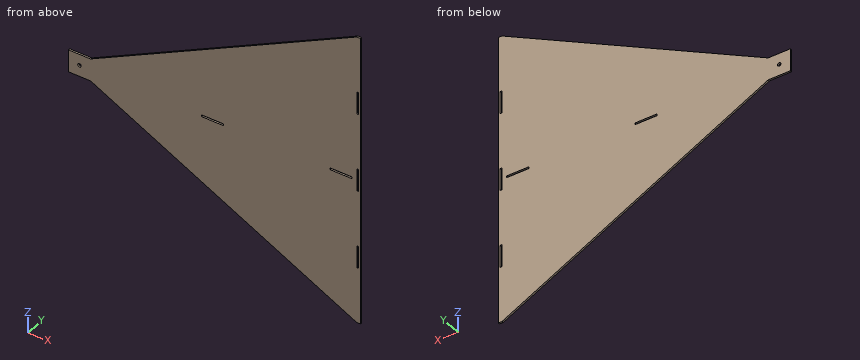
Autodesk Inventor part; units mm, degrees
ref_plane "YZ Plane" through (0, 0, 0) normal (1, 0, 0) x (0, 1, 0)
ref_plane "XZ Plane" through (0, 0, 0) normal (0, 1, 0) x (-1, 0, 0)
ref_plane "XY Plane" through (0, 0, 0) normal (0, 0, 1) x (1, 0, 0)
sketch "Sketch1" plane through (0, 0, 0) normal (0, 1, 0) x (-1, 0, 0)
  line L0 (0, 260) -> (0, -260)
  line L1 (520, 0) -> (0, 260)
  line L2 (0, -260) -> (520, 0)
  point P0 (0, 0)
  dimension "d1" = 260
  dimension "d2" = 520
extrude "Extrusion1" add sketch "Sketch1" along normal blind 3.175
sketch "Sketch2" plane through (0, 3.175, 0) normal (0, 1, 0) x (1, 0, 0)
  circle A0 centre (-500, 0) radius 3.175
  point P0 (0, 0)
  dimension "d6" = 6.35
extrude "Extrusion2" cut sketch "Sketch2" against normal blind 3.175
sketch "Sketch3" plane through (0, 3.175, 0) normal (0, 1, 0) x (1, 0, 0)
  circle A0 centre (-500, 0) radius 3.175
  line L0 (-500, 0) -> (-480, 0)
  line L1 (-480, 0) -> (-480, -20)
  line L2 (-480, -20) -> (-480, 20)
  line L3 (0, 260) -> (-520, 0)
  line L4 (-480, 20) -> (-520, 0)
  line L5 (-520, 0) -> (-480, -20)
  line L6 (-520, 0) -> (0, -260)
  point P0 (0, 0)
extrude "Extrusion3" cut sketch "Sketch3" against normal blind 3.175
sketch "Sketch4" plane through (0, 3.175, 0) normal (0, 1, 0) x (1, 0, 0)
  line L0 (-480, -20) -> (-480, 20)
  line L1 (-480, -20) -> (-520, -20)
  line L2 (-520, -20) -> (-520, 20)
  line L3 (-520, 20) -> (-480, 20)
  point P0 (0, 0)
  dimension "d11" = 40
extrude "Extrusion4" add sketch "Sketch4" against normal blind 3.175
sketch "Sketch5" plane through (0, 3.175, 0) normal (0, 1, 0) x (1, 0, 0)
  circle A0 centre (-500, 0) radius 3.175
  point P0 (0, 0)
  dimension "d15" = 6.35
extrude "Extrusion5" cut sketch "Sketch5" against normal blind 3.175
sketch "Sketch6" plane through (0, 3.175, 0) normal (0, 1, 0) x (1, 0, 0)
  line L0 (-480, -20) -> (0, -260)
  line L1 (0, -260) -> (50, -260)
  line L2 (50, -260) -> (50, 260)
  line L3 (50, 260) -> (0, 260)
  line L4 (0, 260) -> (0, -260)
  point P0 (0, 0)
extrude "Extrusion6" add sketch "Sketch6" against normal blind 3.175
sketch "Sketch8" plane through (0, 3.175, 0) normal (0, 1, 0) x (1, 0, 0)
  line L0 (0, 260) -> (-480, 20)
  line L1 (-480, -20) -> (0, -260)
  line L2 (3.175, -20) -> (0, -20)
  line L3 (0, -20) -> (0, 20)
  line L4 (0, -20) -> (3.2, -20)
  line L5 (0, 20) -> (3.2, 20)
  line L6 (3.2, 20) -> (3.2, -20)
  line L7 (3.2, 160) -> (3.2, 120)
  line L8 (3.2, 120) -> (0, 120)
  line L9 (0, 120) -> (0, 160)
  line L10 (0, 160) -> (3.2, 160)
  line L11 (3.2, -160) -> (3.2, -120)
  line L12 (3.2, -120) -> (0, -120)
  line L13 (0, -120) -> (0, -160)
  line L14 (0, -160) -> (3.2, -160)
  point P0 (0, 0)
  dimension "d23" = 3.2
  dimension "d24" = 3.2
  dimension "d27" = 40
extrude "Extrusion7" cut sketch "Sketch8" against normal blind 10
sketch "Sketch9" plane through (0, 3.175, 0) normal (0, 1, 0) x (1, 0, 0)
  line L0 (3.2, -120) -> (3.2, -160)
  line L1 (6.4, -260) -> (6.4, 260)
  line L2 (0, 260) -> (50, 260)
  line L3 (6.4, 260) -> (50, 260)
  line L4 (50, 260) -> (50, -260)
  line L5 (50, -260) -> (6.4, -260)
  point P0 (0, 0)
extrude "Extrusion8" cut sketch "Sketch9" against normal blind 10
sketch "Sketch10" plane through (0, 3.175, 0) normal (0, 1, 0) x (1, 0, 0)
  line L0 (-520, 20) -> (-520, -20)
  line L1 (-240, 1.6) -> (-280, 1.6)
  line L2 (-280, 1.6) -> (-280, -1.6)
  line L3 (-280, -1.6) -> (-240, -1.6)
  line L4 (-240, -1.6) -> (-240, 1.6)
  point P0 (0, 0)
  dimension "d38" = 40
  dimension "d39" = 40
extrude "Extrusion9" cut sketch "Sketch10" against normal blind 10
sketch "Sketch11" plane through (0, 3.175, 0) normal (0, 1, 0) x (1, 0, 0)
  line L0 (6.4, 260) -> (6.4, -260)
  line L1 (-8.6, 1.6) -> (-8.6, -1.6)
  line L2 (-8.6, -1.6) -> (-48.6, -1.6)
  line L3 (-48.6, -1.6) -> (-48.6, 1.6)
  line L4 (-48.6, 1.6) -> (-8.6, 1.6)
  point P0 (0, 0)
  dimension "d44" = 40
extrude "Extrusion10" cut sketch "Sketch11" against normal blind 10
properties part number "Trebuchet V1 - Truss"
Here's how the part is built. I have some questions about the finished solid (model axes, mm). Coordinates: 2 decimals unless noted, no trailing zeros. Write each loop counter-clockwise with the first axis right and the second up, starting at its lowest first coordinate (ties: lowest second). Pieces come first, ordered by that corner, then holes.
Item 1: Will these pins go through, and if not, where does the flat tip stop? pin 1 (1.6 mm diameter, centred on x = -33.5, y = 1.5, fed in from +Z); pin 2 (1.6 mm diameter, centred on x = -495, y = 1.5, fed in from +Z).
Item 2: I want a section at A-A on y = 2.1. Count the separate pieces of the cut face and the enclosed holes in it, and give its area (3 significant figures).
Item 3: I want a section at B-B on x = -76. Write out the boundary of the cut face in (y, z) (3 decimals), and give its area (3 significant figures).
Item 4: If I drill on line 1 (X direction, y = 1.7, z = 0) (3 decimals); line 2 (Z direction, x = -500, y = 0.8) (3 decimals); line 3 (Z direction, x = -23.5, y = 0.55), over which ranges is the centre line in solid material (lowest first)?
Item 5: I want a section at C-C on z = 46. Write out the boundary of the cut face in (x, y) (3 decimals), and give its area (3 significant figures).
Findings below:
1. pin 1: stops at z = 243.65
1. pin 2: stops at z = 20
2. separate pieces: 1
2. enclosed holes: 6
2. area: 139,000 mm2
3. outline: (0, -222) - (3.175, -222) - (3.175, 222) - (0, 222) - close
3. area: 1,410 mm2
4. line 1: x = -520 to -503.175, -496.825 to -280, -240 to -48.6, -8.6 to 0, 3.2 to 6.4
4. line 2: z = -20 to -3.175, 3.175 to 20
4. line 3: z = -248.25 to -1.6, 1.6 to 248.25
5. outline: (-428, 0) - (6.4, 0) - (6.4, 3.175) - (-428, 3.175) - close
5. area: 1,380 mm2
